from build123d import *

# Parameters (mm, degrees)
BOSS_EXTRUDE1_DEPTH      = 20
BOSS_EXTRUDE1_DEPTH_BACK = 20
SKETCH1_W                = 20
SKETCH1_H                = 6
BOSS_EXTRUDE2_DEPTH      = 20
SKETCH3_W                = 10
SKETCH3_H                = 15
CUT_EXTRUDE1_DEPTH       = 40
FILLET2_R                = 3


with BuildPart() as part:
    # Sketch1 → Boss-Extrude1 (new, two sides: drawn at the far end of the back side and taken through both)
    with BuildSketch(Plane.XY.offset(-BOSS_EXTRUDE1_DEPTH_BACK)):
        Rectangle(SKETCH1_W, SKETCH1_H)
    extrude(amount=BOSS_EXTRUDE1_DEPTH + BOSS_EXTRUDE1_DEPTH_BACK)

    # Sketch2 → Boss-Extrude2 (add)
    with BuildSketch(Plane(origin=(10, 0, 0), x_dir=(0, 0, -1), z_dir=(1, 0, 0))):
        with BuildLine():
            Line((-20, 13), (-20, 3))
            Line((-20, 3), (-10, 3))
            Line((-10, 3), (-10, 13))
            ThreePointArc((-10, 13), (-15, 8), (-20, 13))
        make_face()
        with BuildLine():
            ThreePointArc((-10, 13), (-15, 18), (-20, 13))
            Line((-20, 13), (-16.5, 13))
            ThreePointArc((-16.5, 13), (-15, 14.5), (-13.5, 13))
            Line((-13.5, 13), (-10, 13))
        make_face()
        with BuildLine():
            Line((-16.5, 13), (-20, 13))
            ThreePointArc((-20, 13), (-15, 8), (-10, 13))
            Line((-10, 13), (-13.5, 13))
            ThreePointArc((-13.5, 13), (-15, 11.5), (-16.5, 13))
        make_face()
        with BuildLine():
            ThreePointArc((20, 13), (15, 18), (10, 13))
            Line((10, 13), (13.5, 13))
            ThreePointArc((13.5, 13), (15, 14.5), (16.5, 13))
            Line((16.5, 13), (20, 13))
        make_face()
        with BuildLine():
            Line((13.5, 13), (10, 13))
            ThreePointArc((10, 13), (15, 8), (20, 13))
            Line((20, 13), (16.5, 13))
            ThreePointArc((16.5, 13), (15, 11.5), (13.5, 13))
        make_face()
        with BuildLine():
            Line((10, 13), (10, 3))
            Line((10, 3), (20, 3))
            Line((20, 3), (20, 13))
            ThreePointArc((20, 13), (15, 8), (10, 13))
        make_face()
    extrude(amount=-BOSS_EXTRUDE2_DEPTH)

    # Sketch3 → Cut-Extrude1 (cut)
    with BuildSketch(Plane.XY.offset(20)):
        with Locations((0, 10.5)):
            Rectangle(SKETCH3_W, SKETCH3_H)
    extrude(amount=-CUT_EXTRUDE1_DEPTH, mode=Mode.SUBTRACT)

    # Fillet2
    fillet2_edges = [part.edges().sort_by_distance(p)[0] for p in [
        (0, -3, 20),
        (0, -3, -20),
        (10, -3, 0),
        (-10, -3, 0),
    ]]
    fillet(fillet2_edges, radius=FILLET2_R)


solid = part.part
Design review of the part built by this model. Coordinates are the model's own, in mm. A direction names the side the tool comes from. Give positions to 0.01 mm unless a question says otherwise; leave off trailing zeros. Loops run counter-clockwise (first coordinate to the right, second up) from the corner with the lowest first, then second, coordinate; pieces in that order, holes last. Notation, with made-up numbers: (45.5, 49.5) - (53.5, 49.5) arc R19 cw to (53.5, 76.5) - close; hole circle Ø5 at (-20.75, -40). An arc over 180 degrees is marked (long way). Write item = value, one per line.
1) Tool access review of faces 1 (the face through (-7.46, 12.93, 16.5)), 2 (the face through (-7, 8, -10)), 3 (the face through (5, 10, -15)): name each direction out of +Z, -Z, +X, -X, +Y, -Y from which nothing blocks a thin tool from reaching the whole face with its end or side.
Result sheet:
face_1 = +X, -X
face_2 = +X, -X, +Y
face_3 = +Z, -Z, +Y
2) Take a section at D-D on z = 1.5. State the section outline as (x, y) points.
Result sheet:
outline = (-10, 0) arc R3 ccw to (-7, -3) - (7, -3) arc R3 ccw to (10, 0) - (10, 3) - (-10, 3) - close
3) Draft analysis for pull direction X (two halves, no side actions). For faces 4 (the face through (8, 18, 15)), 5 (the face through (-5, 10, 15)), 6 (the face through (9.1, -2.14, 0.28)), state which applies: +X half, -X half, draft (parallel to the pull), parting line (faces both ways), or undercut.
Result sheet:
face_4 = draft
face_5 = undercut
face_6 = +X half
4) Take a section at A-A on y = 9.75. State the section outline as (x, z) points, and give its area (3 significant figures).
Result sheet:
outline = (-10, -20) - (-5, -20) - (-5, -10) - (-10, -10) - close; (-10, 10) - (-5, 10) - (-5, 20) - (-10, 20) - close; (5, -20) - (10, -20) - (10, -10) - (5, -10) - close; (5, 10) - (10, 10) - (10, 20) - (5, 20) - close
area = 200 mm2
5) To check wall thickness, follow line 1 (Z direction, x = -6.8, y = 13); line 2 (X direction, y = 16.5, z = -14); line 3 (Z direction, x = -5.75, y = 10). State the ranges of each line that lie inside material, in increasing order.
Result sheet:
line_1 = -20 to -16.5, -13.5 to -10, 10 to 13.5, 16.5 to 20
line_2 = -10 to -5, 5 to 10
line_3 = -20 to -10, 10 to 20
6) Clearance check with flat-ended pins moving along their axes: pin 1 Ø1 at (x, z) = (2, 3.5) entering from +Y; pin 2 Ø1.8 at (y, z) = (13, 15) entering from -X. State where each tip first meets the part, or that it passes through.
Result sheet:
pin_1 = 3
pin_2 = through
7) Take a section at B-B on z = 15. State the section outline as (x, y) points, and give its area (3 significant figures).
Result sheet:
outline = (-10, 0) arc R3 ccw to (-7, -3) - (7, -3) arc R3 ccw to (10, 0) - (10, 11.5) - (5, 11.5) - (5, 3) - (-5, 3) - (-5, 11.5) - (-10, 11.5) - close; (-10, 14.5) - (-5, 14.5) - (-5, 18) - (-10, 18) - close; (5, 14.5) - (10, 14.5) - (10, 18) - (5, 18) - close
area = 236 mm2
8) Take a section at C-C on x = 7.5. State the section outline as (y, z) points.
Result sheet:
outline = (-2.96, -17.5) arc R3 ccw to (0, -20) - (13, -20) arc R5 ccw to (13, -10) - (3, -10) - (3, 10) - (13, 10) arc R5 ccw to (13, 20) - (0, 20) arc R3 ccw to (-2.96, 17.5) - close; hole circle Ø3 at (13, -15); hole circle Ø3 at (13, 15)
